from build123d import *

# Parameters (mm, degrees)
F0_R     = 3
F1_DEPTH = 50
F2_R     = 1
F4_W     = 9.6827019006
F4_H     = 44
F5_DEPTH = 2
F7_D     = 2.5


with BuildPart() as f1:
    # F0 (on Top) → F1 (new body)
    with BuildSketch(Plane.XY):
        Circle(F0_R)
    extrude(amount=F1_DEPTH)

    # F2
    f2_edges = [f1.edges().sort_by_distance(p)[0] for p in [
        (-3, 0, 50),
    ]]
    fillet(f2_edges, radius=F2_R)

    # F4 (on offset) → F5 (cut)
    with BuildSketch(Plane.YZ.offset(3)):
        Rectangle(F4_W, F4_H)
    extrude(amount=-F5_DEPTH, mode=Mode.SUBTRACT)

    # F7 (through all)
    with Locations(Plane.YZ.offset(1)):
        with Locations((0, 3.5), (0, 18.5)):
            Hole(F7_D / 2)


solid = f1.part
CAD build for the part. Positions are in the model's coordinates, mm. A direction names the side the tool comes from. Give positions to 0.01 mm unless a question says otherwise; leave off trailing zeros. Order: outer loops, then holes, each group sorted by start corner. A loop starts at its lowest first (then second) coordinate and runs counter-clockwise, first axis right, second up. Notation, with made-up numbers: (-14, -11.75) -> (27, -11.75) arc R20 cw to (27, 25.25) -> close; hole circle Ø3 at (30.5, 65). An arc over 180 degrees is marked (long way). Return JSON: item names as keys, results as strings.
Q1. Flat gauge pins, fed straight in: pin 1 (3 mm diameter, centred on y = 2, z = 12, fed in from -X); pin 2 (3 mm diameter, centred on y = 1.5, z = 15.5, fed in from +X); pin 3 (1.5 mm diameter, centred on y = 0, z = 18.5, fed in from -X). Where does each tip first touch, or does it go through?
Working result:
{"pin 1": "x = -2.96", "pin 2": "x = 1", "pin 3": "through"}
Q2. Mould opens along Y. For faces 1 (the face through (2, 0, 22)), 2 (the face through (-1.03, 1.25, 18.55)), 3 (the face through (-3, 0, 30)) say: pulls with the +Y half, pulls with the -Y half, needs draft (parallel to the pull), parting line crosses it, or undercut.
Working result:
{"face 1": "needs draft", "face 2": "undercut", "face 3": "parting line crosses it"}
Q3. Saw through at D-D (x = 0.5). Count the separate pieces of the cut face and the enclosed holes in it, then the cut area to 3 significant figures.
Working result:
{"separate pieces": "1", "enclosed holes": "2", "area": "286 mm²"}
Q4. Saw through at B-B (z = 18.5). Write the cut outline in (x, y).
Working result:
{"outline": "(-2.73, -1.25) arc R3 ccw to (1, -2.83) -> (1, -1.25) -> close; (-2.73, 1.25) -> (1, 1.25) -> (1, 2.83) arc R3 ccw to start"}
Q5. Which spindle directions (+Z, -Z, +X, -X, +Y, -Y) get a long thin tool onto all of the face, cutting with end or side? Do faces 4 (the face through (1, 0, 11)), 5 (the face through (-1, 0, 0)). Say none if no direction does.
Working result:
{"face 4": "-Z, +X, +Y, -Y", "face 5": "-Z, +X, -X, +Y, -Y"}
Q6. Drill centre lines: line 1 (Z direction, x = -0.2, y = 0); line 2 (X direction, y = -1, z = 6.5); line 3 (Y direction, x = -1.45, z = 3.5). Where is each one in solid material? Low to high.
Working result:
{"line 1": "0 to 2.25, 4.75 to 17.25, 19.75 to 50", "line 2": "-2.83 to 1", "line 3": "-2.63 to -1.25, 1.25 to 2.63"}
Q7. Saw through at A-A (y = 0). Write the cut outline in (x, z), then the cut area to 3 significant figures.
Working result:
{"outline": "(-3, 0) -> (1, 0) -> (1, 2.25) -> (-3, 2.25) -> close; (-3, 4.75) -> (1, 4.75) -> (1, 17.25) -> (-3, 17.25) -> close; (-3, 19.75) -> (1, 19.75) -> (1, 22) -> (3, 22) -> (3, 49) arc R1 ccw to (2, 50) -> (-2, 50) arc R1 ccw to (-3, 49) -> close", "area": "236 mm²"}
Q8. Saw through at C-C (z = 28.5). Write the cut outline in (x, y), then the cut area to 3 significant figures.
Working result:
{"outline": "circle Ø6 at (0, 0)", "area": "28.3 mm²"}
